Design review of the part built by this model. Coordinates are the model's own, in mm. Face numbers are marked on the shaded views. Give positions to 0.01 mm unless a question says otherwise; leave off trailing zeros. Loops run counter-clockwise (first coordinate to the right, second up) from the corner with the lowest first, then second, coordinate; pieces in that order, holes last. Notation, with made-up numbers: (31.25, 89) -> (74.25, 89) arc R18 cw to (74.25, 100) -> close; hole circle Ø2 at (79, -9). An arc over 180 degrees is marked (long way). Use a Markdown table: item, result. Add a question column.
1. For pin 1 Ø1 at (x, z) = (5.5, 1) entering from +Y; pin 2 Ø0.9 at (y, z) = (0.5, 1) entering from -X, all flat-tipped, find the tip position at first contact; note any pin that passes through.
2. To check wall thickness, follow line 1 (Z direction, x = 6, y = 0.25); line 2 (Z direction, x = 2.75, y = 0.4); line 3 (X direction, y = 1.85, z = 0.7). State the ranges of each line that lie inside material, in increasing order.
3. Add section A-A (y = 0.5). State the section outline as (x, z) points, and give its area (3 significant figures).
4. Add section B-B (x = 6.25). State the section outline as (y, z) points.
5. Add section C-C (y = 1.7). State the section outline as (x, z) points, and give its area (3 significant figures).
6. Draft analysis for pull direction Z (two halves, no side actions). For the marked faces 1, 2 and 3, state which applies: pulls with the +Z half, pulls with the -Z half, needs draft (parallel to the pull), parting line crosses it, or undercut.
7. Add section D-D (z = 0.9). State the section outline as (x, y) points.
```python
from build123d import *

# Parameters (mm, degrees)
EXTRUDE_1_DEPTH = 0.25
SKETCH_2_W      = 4.8
SKETCH_2_H      = 0.25
EXTRUDE_2_DEPTH = 0.95
SKETCH_3_W      = 0.25
SKETCH_3_H      = 1.95
EXTRUDE_3_DEPTH = 2.068252296
SKETCH_4_W      = 0.25
SKETCH_4_H      = 1.95
EXTRUDE_4_DEPTH = 0.668252296
FILLET_1_R      = 0.5
FILLET_2_R      = 0.75


with BuildPart() as part:
    # 草图1 → 凸台-拉伸1 (new body)
    with BuildSketch(Plane(origin=(0, 0, -0.25), x_dir=(-1, 0, 0), z_dir=(0, 0, -1))):
        with BuildLine():
            Line((0.486013986, 1), (-6.813986014, 1))
            Line((-6.813986014, 1), (-6.813986014, 0))
            Line((-6.813986014, 0), (0.486013986, 0))
            ThreePointArc((0.486013986, 0), (0.986013986, 0.5), (0.486013986, 1))
        make_face()
    extrude(amount=-EXTRUDE_1_DEPTH)

    # 草图2 → 凸台-拉伸2 (add)
    with BuildSketch(Plane(origin=(0, 1, 0), x_dir=(-1, 0, 0), z_dir=(0, 1, 0))):
        with Locations((-4.413986014, -0.125)):
            Rectangle(SKETCH_2_W, SKETCH_2_H)
    extrude(amount=EXTRUDE_2_DEPTH)

    # 草图3 → 凸台-拉伸3 (add)
    with BuildSketch(Plane.XY):
        with Locations((6.688986014, 0.975)):
            Rectangle(SKETCH_3_W, SKETCH_3_H)
    extrude(amount=EXTRUDE_3_DEPTH)

    # 草图4 → 凸台-拉伸4 (add)
    with BuildSketch(Plane.ZY.offset(-6.563986014)):
        with Locations((1.943252296, 0.975)):
            Rectangle(SKETCH_4_W, SKETCH_4_H)
    extrude(amount=EXTRUDE_4_DEPTH)

    # 圆角1
    fillet_1_edges = [part.edges().sort_by_distance(p)[0] for p in [
        (6.563986014, 0.975, 0),
        (6.563986014, 0.975, 1.818252296),
    ]]
    fillet(fillet_1_edges, radius=FILLET_1_R)

    # 圆角2
    fillet_2_edges = [part.edges().sort_by_distance(p)[0] for p in [
        (6.813986014, 0.975, 2.068252296),
        (6.813986014, 0.975, -0.25),
    ]]
    fillet(fillet_2_edges, radius=FILLET_2_R)


solid = part.part
```
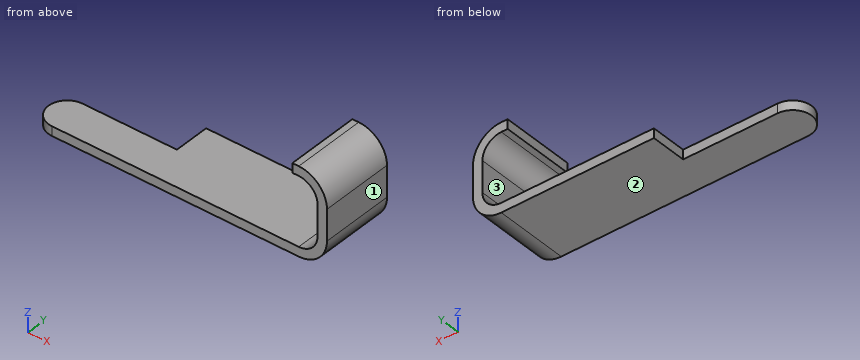
Taken from the geometry:
| question | item | result |
|---|---|---|
| 1 | pin 1 | passes through |
| 1 | pin 2 | stops at x = 6.55 |
| 2 | line 1 | z = -0.25 to 0, 1.82 to 2.07 |
| 2 | line 2 | z = -0.25 to 0 |
| 2 | line 3 | x = 6.56 to 6.81 |
| 3 | outline | (-0.99, -0.25) -> (6.06, -0.25) arc R0.75 ccw to (6.81, 0.5) -> (6.81, 1.32) arc R0.75 ccw to (6.06, 2.07) -> (5.9, 2.07) -> (5.9, 1.82) -> (6.06, 1.82) arc R0.5 cw to (6.56, 1.32) -> (6.56, 0.5) arc R0.5 cw to (6.06, 0) -> (-0.99, 0) -> close |
| 3 | area | 2.50 mm^2 |
| 4 | outline | (0, -0.23) -> (1.95, -0.23) -> (1.95, 0.04) -> (0, 0.04) -> close; (0, 1.78) -> (1.95, 1.78) -> (1.95, 2.04) -> (0, 2.04) -> close |
| 5 | outline | (2.01, -0.25) -> (6.06, -0.25) arc R0.75 ccw to (6.81, 0.5) -> (6.81, 1.32) arc R0.75 ccw to (6.06, 2.07) -> (5.9, 2.07) -> (5.9, 1.82) -> (6.06, 1.82) arc R0.5 cw to (6.56, 1.32) -> (6.56, 0.5) arc R0.5 cw to (6.06, 0) -> (2.01, 0) -> close |
| 5 | area | 1.75 mm^2 |
| 6 | face 1 | needs draft |
| 6 | face 2 | pulls with the -Z half |
| 6 | face 3 | undercut |
| 7 | outline | (6.56, 0) -> (6.81, 0) -> (6.81, 1.95) -> (6.56, 1.95) -> close |
